Check sheet for the modelled part. Datum: model origin and axes. Units: mm. Face numbers are marked on the shaded views. A direction names the side the tool comes from. Round coordinates to 2 decimals unless told otherwise and drop trailing zeros. Order: outer loops, then holes, each group sorted by start corner. A loop starts at its lowest first (then second) coordinate and runs counter-clockwise, first axis right, second up.
Q1. Cross-section at A-A on y = 23. Record the cut outline in (x, z) (3 decimals).
Q2. Depth check by flat-ended pin: P1, Ø6, axis at x = 81, y = 26, coming from the +Z side; P2, Ø12, axis at y = 14, z = -14.5, coming from the -X side; P3, Ø1, axis at x = 93.5, y = 8, coming from the -Z side. Enter the tip coordinate at first touch or a pass-through.
Q3. Cross-section at B-B on z = -59.5. Record the cut outline in (x, y) (3 decimals).
Q4. Mould release check, pull along X, two halves, no side actions. Record for the marked faces 1, 2 and 3: +X half, -X half, draft (parallel to the pull), parting line (faces both ways), or undercut.
Q5. Cross-section at D-D on x = 36. Record the cut outline in (y, z) (3 decimals), then the cut area to 3 significant figures.
Q6. Scan lines: probe 1 along Z at (x, y) = (57, 30) (3 decimals); probe 2 along X at (y, z) = (27.5, -68.5); probe 3 along X at (y, z) = (35, -21.5) (3 decimals). Record each from-to range of solid material in increasing order.
Q7. Set-up check for the marked faces 4, 5, 6 and 7: record each of +Z, -Z, +X, -X, +Y, -Y from which the full face is reachable in a straight line by a thin tool's end or side.
Q8. Cross-section at C-C on y = 17. Record the cut outline in (x, z) (3 decimals).
from build123d import *

# Parameters (mm, degrees)
SKETCH1_W           = 95.25
SKETCH1_H           = 69.85
BOSS_EXTRUDE1_DEPTH = 38.1
SKETCH2_W           = 88.9
SKETCH2_H           = 63.5
CUT_EXTRUDE1_DEPTH  = 31.75
CUT_EXTRUDE2_REACH  = 126.11
SKETCH3_W           = 6.35
SKETCH3_H           = 3.81
CUT_EXTRUDE3_REACH  = 126.11
SKETCH4_W           = 15.24
SKETCH4_H           = 10.16
SKETCH5_W           = 100.33
SKETCH5_H           = 74.93
BOSS_EXTRUDE2_DEPTH = 2.54
SKETCH6_W           = 11.43
SKETCH6_H           = 10.929541263
CUT_EXTRUDE4_DEPTH  = 6.35
SKETCH7_W           = 14.362267298
SKETCH7_H           = 6.50180408
CUT_EXTRUDE5_DEPTH  = 6.35


with BuildPart() as part:
    # Sketch1 → Boss-Extrude1 (new body)
    with BuildSketch(Plane(origin=(0, 0, 0), x_dir=(1, 0, 0), z_dir=(0, 1, 0))):
        with Locations((47.625, 34.925)):
            Rectangle(SKETCH1_W, SKETCH1_H)
    extrude(amount=BOSS_EXTRUDE1_DEPTH)

    # Sketch2 → Cut-Extrude1 (cut)
    with BuildSketch(Plane(origin=(0, 38.1, 0), x_dir=(1, 0, 0), z_dir=(0, 1, 0))):
        with Locations((47.625, 34.925)):
            Rectangle(SKETCH2_W, SKETCH2_H)
    extrude(amount=-CUT_EXTRUDE1_DEPTH, mode=Mode.SUBTRACT)

    # Sketch3 → Cut-Extrude2 (cut, up to next)
    with BuildSketch(Plane(origin=(95.25, 0, 0), x_dir=(0, 0, -1), z_dir=(1, 0, 0)), mode=Mode.PRIVATE) as cut_extrude2_sk1:
        with Locations((59.69, 10.795)):
            Rectangle(SKETCH3_W, SKETCH3_H)
    cut_extrude2_tool1 = extrude(cut_extrude2_sk1.sketch, amount=-CUT_EXTRUDE2_REACH, mode=Mode.PRIVATE) & part.part
    add(cut_extrude2_tool1.solids().sort_by_distance((95.25, 10.795, -59.69))[0], mode=Mode.SUBTRACT)

    # Sketch4 → Cut-Extrude3 (cut, up to next)
    with BuildSketch(Plane.ZY, mode=Mode.PRIVATE) as cut_extrude3_sk1:
        with Locations((-14.605, 24.13)):
            Rectangle(SKETCH4_W, SKETCH4_H)
    cut_extrude3_tool1 = extrude(cut_extrude3_sk1.sketch, amount=-CUT_EXTRUDE3_REACH, mode=Mode.PRIVATE) & part.part
    add(cut_extrude3_tool1.solids().sort_by_distance((0, 24.13, -14.605))[0], mode=Mode.SUBTRACT)

    # Sketch5 → Boss-Extrude2 (add)
    with BuildSketch(Plane.XZ):
        with Locations((47.625, -34.925)):
            Rectangle(SKETCH5_W, SKETCH5_H)
    extrude(amount=-BOSS_EXTRUDE2_DEPTH)

    # Sketch6 → Cut-Extrude4 (cut)
    with BuildSketch(Plane(origin=(0, 0, -69.85), x_dir=(-1, 0, 0), z_dir=(0, 0, -1))):
        with Locations((-47.879, 26.743022326)):
            Rectangle(SKETCH6_W, SKETCH6_H)
    extrude(amount=-CUT_EXTRUDE4_DEPTH, mode=Mode.SUBTRACT)

    # Sketch7 → Cut-Extrude5 (cut)
    with BuildSketch(Plane(origin=(95.25, 0, 0), x_dir=(0, 0, -1), z_dir=(1, 0, 0))):
        with Locations((32.45447078, 9.60090204)):
            Rectangle(SKETCH7_W, SKETCH7_H)
    extrude(amount=-CUT_EXTRUDE5_DEPTH, mode=Mode.SUBTRACT)


solid = part.part
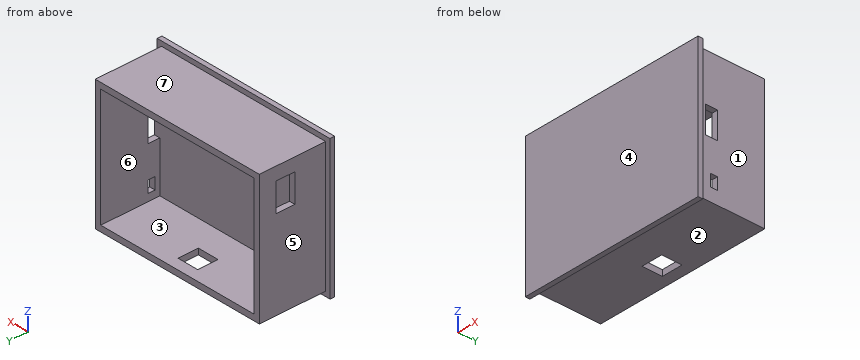
Results found:
1. outline: (0, -69.85) - (42.164, -69.85) - (42.164, -66.675) - (3.175, -66.675) - (3.175, -22.225) - (0, -22.225) - close; (0, -6.985) - (3.175, -6.985) - (3.175, -3.175) - (92.075, -3.175) - (92.075, -66.675) - (53.594, -66.675) - (53.594, -69.85) - (95.25, -69.85) - (95.25, 0) - (0, 0) - close
2. P1: stops at z = 0
2. P2: stops at x = 0
2. P3: stops at z = -69.85
3. outline: (-2.54, 0) - (97.79, 0) - (97.79, 2.54) - (95.25, 2.54) - (95.25, 8.89) - (92.075, 8.89) - (92.075, 6.35) - (3.175, 6.35) - (3.175, 38.1) - (0, 38.1) - (0, 2.54) - (-2.54, 2.54) - close; (92.075, 12.7) - (95.25, 12.7) - (95.25, 38.1) - (92.075, 38.1) - close
4. face 1: +X half
4. face 2: draft
4. face 3: undercut
5. outline: (0, -72.39) - (2.54, -72.39) - (2.54, -69.85) - (38.1, -69.85) - (38.1, -66.675) - (6.35, -66.675) - (6.35, -3.175) - (38.1, -3.175) - (38.1, 0) - (2.54, 0) - (2.54, 2.54) - (0, 2.54) - close
5. area: 658 mm2
6. probe 1: z = -69.85 to -66.675, -3.175 to 0
6. probe 2: x = 0 to 42.16, 53.59 to 95.25
6. probe 3: x = 0 to 3.175, 92.075 to 95.25
7. face 4: +Z, -Z, +X, -X, -Y
7. face 5: +Z, -Z, -X, +Y
7. face 6: +Y
7. face 7: +Z, +X, -X, +Y
8. outline: (0, -69.85) - (95.25, -69.85) - (95.25, 0) - (0, 0) - close; hole (3.175, -66.675) - (92.075, -66.675) - (92.075, -3.175) - (3.175, -3.175) - close
